```python
from build123d import *

# Parameters (mm, degrees)
F0_R     = 1.2446
F0_R_2   = 8.636
F1_DEPTH = 8.89
F0_R_3   = 8.509
F2_DEPTH = 3.175


with BuildPart() as f1:
    # F0 (on Front) → F1 (new body)
    with BuildSketch(Plane.XZ):
        with BuildLine():
            Line((6.6421, 9.906), (-6.6421, 9.906))
            ThreePointArc((-6.6421, 9.906), (-11.132228, 8.046128), (-12.9921, 3.556))
            Line((-12.9921, 3.556), (-12.9921, 1.524))
            ThreePointArc((-12.9921, 1.524), (-9.644331, -6.558231), (-1.5621, -9.906))
            Line((-1.5621, -9.906), (1.5621, -9.906))
            ThreePointArc((1.5621, -9.906), (9.644331, -6.558231), (12.9921, 1.524))
            Line((12.9921, 1.524), (12.9921, 3.556))
            ThreePointArc((12.9921, 3.556), (11.132228, 8.046128), (6.6421, 9.906))
        make_face()
        with Locations((-10.4775, 0)):
            Circle(F0_R, mode=Mode.SUBTRACT)
        Circle(F0_R_2, mode=Mode.SUBTRACT)
        with Locations((10.4775, 0)):
            Circle(F0_R, mode=Mode.SUBTRACT)
    extrude(amount=F1_DEPTH)

    # F0 (on Front) → F2 (join)
    with BuildSketch(Plane.XZ):
        Circle(F0_R_2)
        Circle(F0_R_3, mode=Mode.SUBTRACT)
    extrude(amount=F2_DEPTH)


solid = f1.part
```
Geometry: final body of the model. Coordinates: model frame, mm. Round coordinates to 2 decimals unless told otherwise and drop trailing zeros. Order: outer loops, then holes, each group sorted by start corner. A loop starts at its lowest first (then second) coordinate and runs counter-clockwise, first axis right, second up. Notation, with made-up numbers: (67.25, -29) - (115.25, -29) arc R19 ccw to (115.25, -17) - close; hole circle Ø10 at (-24, 12.5). An arc over 180 degrees is marked (long way). Use CSV: the item, a comma, the result in double quotes. Start each with the question number.
Q1. Section query D-D (z = 0). Return loops of the section in (x, y) (3 decimals), and give its area (3 significant figures).
Q2. Section query A-A (y = -7). Return loops of the section in (x, z).
Q3. Section query B-B (z = -7). Return loops of the section in (x, y) (3 decimals), and give its area (3 significant figures).
Q4. First-contact query: pin 1 (5 mm diameter, centred on y = -3.5, z = -4.5, fed in from +X); pin 2 (2 mm diameter, centred on x = 10.48, z = 0, fed in from -Y); pin 3 (1.5 mm diameter, centred on x = -3, y = -1.5, fed in from -Z). Flat tips, straight axial feed; report the tip coordinate or a pass-through.
Q5. Section query C-C (x = 0). Return loops of the section in (y, z) (3 decimals), and give its area (3 significant figures).
Q6. Mould query, pull axis Z, two halves, no side actions, for faces 1 (the face through (-11.08, -4.38, 8.1)), 2 (the face through (-1.124, -5.992, 8.563)), 3 (the face through (-6, -8.89, 7)). Classes: +Z half, -Z half, draft (parallel to the pull), parting line (faces both ways), or undercut.
Q7. Material intervals for line 1 along Z through (x, y) = (1.5, -6.75); line 2 along X through (y, z) = (-2.25, -1); line 3 along X through (y, z) = (-3.5, 0.5), sorted ascending. Write a range as from..to.
Result set:
1,outline,"(-12.89, -8.89) - (-11.722, -8.89) - (-11.722, 0) - (-12.89, 0) - close; (-9.233, -8.89) - (-8.636, -8.89) - (-8.636, -3.175) - (-8.509, -3.175) - (-8.509, 0) - (-9.233, 0) - close; (8.509, -3.175) - (8.636, -3.175) - (8.636, -8.89) - (9.233, -8.89) - (9.233, 0) - (8.509, 0) - close; (11.722, -8.89) - (12.89, -8.89) - (12.89, 0) - (11.722, 0) - close"
1,area,"32.2 mm2"
2,outline,"(-12.99, 1.52) arc R11.43 ccw to (-1.56, -9.91) - (1.56, -9.91) arc R11.43 ccw to (12.99, 1.52) - (12.99, 3.56) arc R6.35 ccw to (6.64, 9.91) - (-6.64, 9.91) arc R6.35 ccw to (-12.99, 3.56) - close; hole circle Ø2.49 at (-10.48, 0); hole circle Ø17.27 at (0, 0); hole circle Ø2.49 at (10.48, 0)"
3,outline,"(-9.177, -8.89) - (-5.058, -8.89) - (-5.058, -3.175) - (-4.838, -3.175) - (-4.838, 0) - (-9.177, 0) - close; (4.838, -3.175) - (5.058, -3.175) - (5.058, -8.89) - (9.177, -8.89) - (9.177, 0) - (4.838, 0) - close"
3,area,"74.6 mm2"
4,pin 1,"stops at x = 12.44"
4,pin 2,"passes through"
4,pin 3,"stops at z = -9.89"
5,outline,"(-8.89, -9.906) - (0, -9.906) - (0, -8.509) - (-3.175, -8.509) - (-3.175, -8.636) - (-8.89, -8.636) - close; (-8.89, 8.636) - (-3.175, 8.636) - (-3.175, 8.509) - (0, 8.509) - (0, 9.906) - (-8.89, 9.906) - close"
5,area,"23.4 mm2"
6,face 1,"+Z half"
6,face 2,"undercut"
6,face 3,"draft"
7,line 1,"z = -9.91..-8.5, 8.5..9.91"
7,line 2,"x = -12.71..-11.22, -9.74..-8.45, 8.45..9.74, 11.22..12.71"
7,line 3,"x = -12.95..-11.62, -9.34..-8.62, 8.62..9.34, 11.62..12.95"
